Job drawing, mm, ordinate dimensions from the low corner. One solid piece. A direction names the side the tool comes from. Give positions to 0.01 mm unless a question says otherwise; leave off trailing zeros. Write each loop counter-clockwise with the first axis right and the second up, starting at its lowest first coordinate (ties: lowest second). Pieces come first, ordered by that corner, then holes. Notation, with made-up numbers: (88, -24) - (137, -24) arc R27 cw to (137, 1) - close; hole circle Ø5 at (39.5, 3). An arc over 180 degrees is marked (long way). Answer in a Markdown table with one row per item. Add a question column.
1. Pull direction Z, two halves, no side cores. Call the marked faces 1, 2 and 3: released by +Z, released by -Z, zero draft, split by the parting line, or undercut.
2. Which spindle directions (+Z, -Z, +X, -X, +Y, -Y) get a long thin tool onto all of the face, cutting with end or side? Do the marked faces 4 and 5. Say none if no direction does.
3. Band-saw the part on B-B on z = 8.75. Write the cut outline in (x, y), plus the area to 3 significant figures.
4. Band-saw the part on C-C on y = 9. Write the cut outline in (x, z).
5. Probe line 1 along Z through (x, y) = (9, 2.3); line 2 along Y through (x, z) = (9, 2.8); line 3 along Y through (x, z) = (7.25, 4.5). List the from-to ranges inside material, lowest first.
6. Band-saw the part on D-D on z = 3.75. Write the cut outline in (x, y).
7. Drop flat-ended pins along their axis: pin 1 Ø9 at (x, y) = (9, 9) entering from -Z; pin 2 Ø5 at (y, z) = (2, 6.5) entering from +X; pin 3 Ø1 at (y, z) = (5, 6.5) entering from +X. Give the stop position or say it passes through.
8. Band-saw the part on A-A on x = 9. Write the cut outline in (y, z).
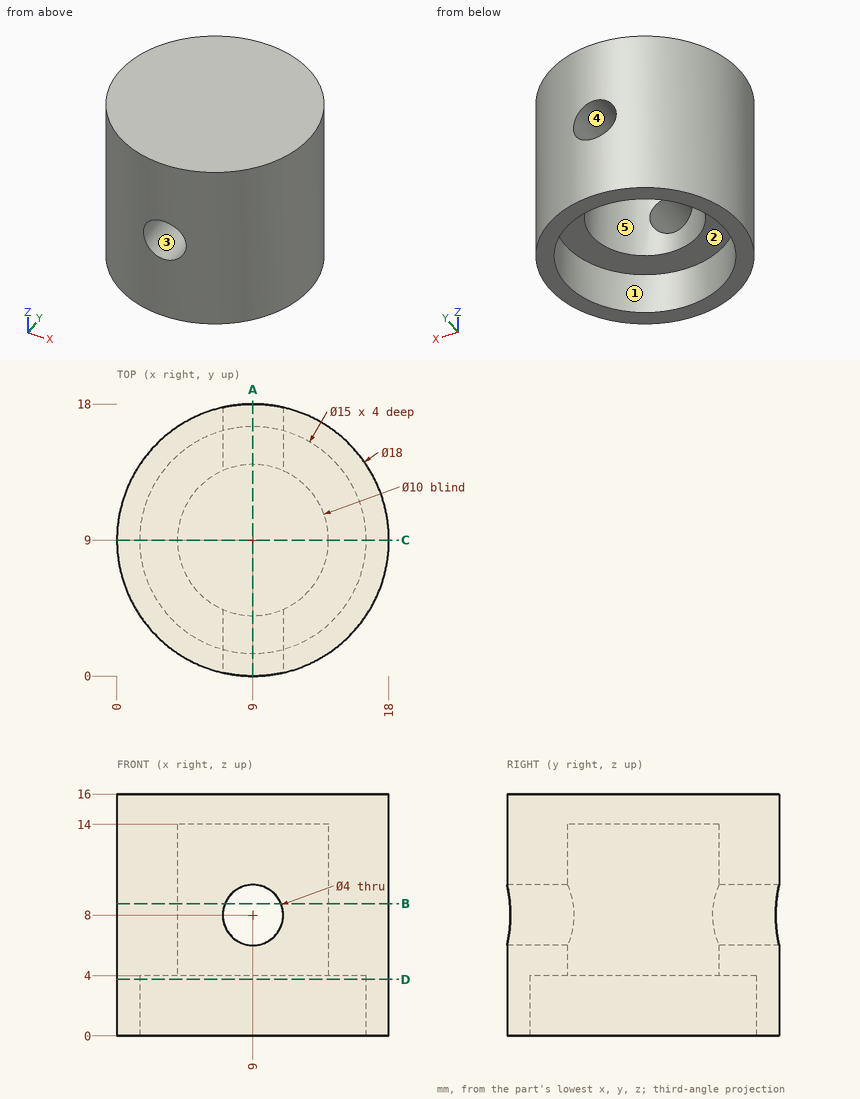
Values:
| question | item | result |
|---|---|---|
| 1 | face 1 | zero draft |
| 1 | face 2 | released by -Z |
| 1 | face 3 | undercut |
| 2 | face 4 | +Y, -Y |
| 2 | face 5 | -Z |
| 3 | outline | (7.15, 0.19) - (7.15, 4.36) arc R5 cw to (7.15, 13.64) - (7.15, 17.81) arc R9 ccw to start; (10.85, 0.19) arc R9 ccw to (10.85, 17.81) - (10.85, 13.64) arc R5 cw to (10.85, 4.36) - close |
| 3 | area | 146 mm² |
| 4 | outline | (0, 0) - (1.5, 0) - (1.5, 4) - (4, 4) - (4, 14) - (14, 14) - (14, 4) - (16.5, 4) - (16.5, 0) - (18, 0) - (18, 16) - (0, 16) - close |
| 5 | line 1 | z = 4 to 6, 10 to 16 |
| 5 | line 2 | y = 0 to 1.5, 16.5 to 18 |
| 5 | line 3 | y = 0.17 to 4.32, 13.68 to 17.83 |
| 6 | outline | circle Ø18 at (9, 9); hole circle Ø15 at (9, 9) |
| 7 | pin 1 | stops at z = 14 |
| 7 | pin 2 | stops at x = 16.79 |
| 7 | pin 3 | stops at x = 17.29 |
| 8 | outline | (0, 0) - (1.5, 0) - (1.5, 4) - (4, 4) - (4, 6) - (0, 6) - close; (0, 10) - (4, 10) - (4, 14) - (14, 14) - (14, 10) - (18, 10) - (18, 16) - (0, 16) - close; (14, 4) - (16.5, 4) - (16.5, 0) - (18, 0) - (18, 6) - (14, 6) - close |
